Could you check a few things on this drawing? It's one solid part, dimensions in mm from its lowest x, y, z. A direction names the side the tool comes from. Give positions to 0.01 mm unless a question says otherwise; leave off trailing zeros. Order: outer loops, then holes, each group sorted by start corner. A loop starts at its lowest first (then second) coordinate and runs counter-clockwise, first axis right, second up.
Item 1: I want a section at A-A, the plane x = 1. Write out the boundary of the cut face in (y, z).
Item 2: If I drill on line 1 along Y through (x, z) = (4, 49.5); line 2 along Y through (x, z) = (0.5, 37.5); line 3 along X through (y, z) = (30, 46.5), over which ranges is the centre line in solid material (lowest first)?
Item 3: Which directions (+Z, -Z, +X, -X, +Y, -Y) give clear straight access to the entire face, cutting with the end or side of a thin tool? Please do the marked faces 1 and 2.
Item 4: I'm going to push flat-ended pins straight in: pin 1 Ø3 at (x, z) = (4, 29) entering from -Y; pin 2 Ø2 at (y, z) = (13, 48.5) entering from +X; pin 3 Ø1 at (x, z) = (6, 42) entering from +Y. Where does each tip first touch, or does it pass through?
Item 5: I want a section at D-D, the plane y = 27. Write out the boundary of the cut face in (x, z), then the cut area to 3 significant figures.
Item 6: I want a section at C-C, the plane x = 6. Write out the boundary of the cut face in (y, z).
Item 7: I want a section at B-B, the plane z = 50. Write out the boundary of the cut face in (x, y).
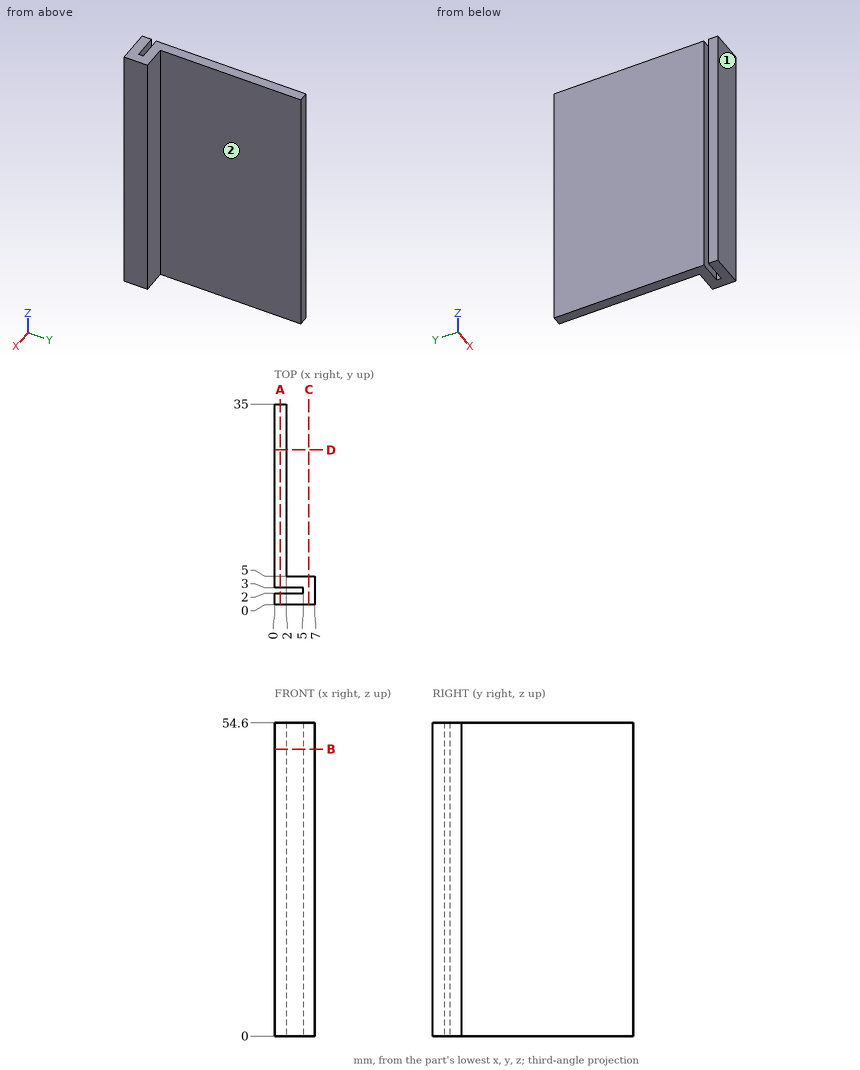
Results list:
1. outline: (0, 0) - (2, 0) - (2, 54.6) - (0, 54.6) - close; (3, 0) - (35, 0) - (35, 54.6) - (3, 54.6) - close
2. line 1: y = 0 to 2, 3 to 5
2. line 2: y = 0 to 2, 3 to 35
2. line 3: x = 0 to 2
3. face 1: +Z, -Z, +X, -X, -Y
3. face 2: +Z, -Z, +X, +Y
4. pin 1: stops at y = 0
4. pin 2: stops at x = 2
4. pin 3: stops at y = 5
5. outline: (0, 0) - (2, 0) - (2, 54.6) - (0, 54.6) - close
5. area: 109 mm2
6. outline: (0, 0) - (5, 0) - (5, 54.6) - (0, 54.6) - close
7. outline: (0, 0) - (7, 0) - (7, 5) - (2, 5) - (2, 35) - (0, 35) - (0, 3) - (5, 3) - (5, 2) - (0, 2) - close
